Geometry: final body of the model. Coordinates: model frame, mm. Face numbers are marked on the shaded views. A direction names the side the tool comes from. Give positions to 0.01 mm unless a question says otherwise; leave off trailing zeros. Order: outer loops, then holes, each group sorted by start corner. A loop starts at its lowest first (then second) coordinate and runs counter-clockwise, first axis right, second up. Notation, with made-up numbers: M 84,1.25 L 119,1.25 A19 ccw 119,36.25 Z; hole C -13.5,89 d1. An arc over 180 degrees is marked long. Use CSV: the item, a comma, the result in double quotes.
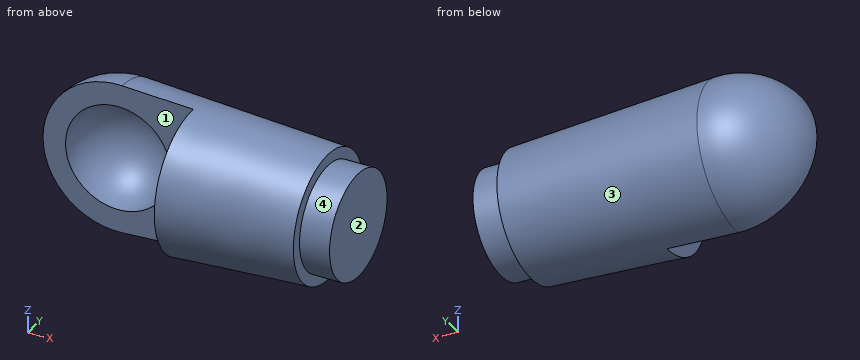
```python
from build123d import *

# Parameters (mm, degrees)
SKETCH2_W           = 100
SKETCH2_H           = 100
CUT_EXTRUDE1_DEPTH  = 62
SKETCH3_R           = 35
BOSS_EXTRUDE1_DEPTH = 20


with BuildPart() as part:
    # Sketch1 → Revolve1 (revolve)
    with BuildSketch(Plane(origin=(0, 0, 0), x_dir=(1, 0, 0), z_dir=(0, 1, 0)), mode=Mode.PRIVATE) as revolve1_sk:
        with BuildLine():
            Line((0, 0), (0, 42.5))
            Line((0, 42.5), (-137.299270073, 49.927007299))
            ThreePointArc((-137.299270073, 49.927007299), (-174.387232396, 36.297634195), (-190, 0))
            Line((-190, 0), (-175, 0))
            ThreePointArc((-175, 0), (-140, 35), (-105, 0))
            Line((-105, 0), (0, 0))
        make_face()
    revolve(revolve1_sk.sketch.rotate(Axis((-105, 0, 0), (1, 0, 0)), 180), axis=Axis((-105, 0, 0), (1, 0, 0)))

    # Sketch2 → Cut-Extrude1 (cut)
    with BuildSketch(Plane(origin=(0, 0, 0), x_dir=(1, 0, 0), z_dir=(0, 1, 0))):
        with Locations((-140, 0)):
            Rectangle(SKETCH2_W, SKETCH2_H)
    extrude(amount=-CUT_EXTRUDE1_DEPTH, mode=Mode.SUBTRACT)

    # Sketch3 → Boss-Extrude1 (add)
    with BuildSketch(Plane(origin=(0, 0, 0), x_dir=(0, 0, -1), z_dir=(1, 0, 0))):
        Circle(SKETCH3_R)
    extrude(amount=BOSS_EXTRUDE1_DEPTH)


solid = part.part
```
1. Pull-direction query (X, two-part tool) for the marked faces 3 and 4; classes: +X half, -X half, draft (parallel to the pull), parting line (faces both ways), or undercut.
Answer:
face 3,"+X half"
face 4,"draft"
2. Section A-A, the plane z = 0. Return the cut outline in (x, y), plus the area to 3 significant figures.
Answer:
outline,"M -190,0 L -175,0 A35 cw -105,0 L -90,0 L -90,-47.37 L 0,-42.5 L 0,-35 L 20,-35 L 20,35 L 0,35 L 0,42.5 L -137.3,49.93 A50 ccw Z"
area,"12,000 mm2"
3. Line query: line 1 (X direction, y = -18, z = 19); line 2 (X direction, y = 23, z = -24.5); line 3 (Z direction, x = -153.5, y = 20.5). Output: solid intervals per line, ascending.
Answer:
line 1,"-90 to 20"
line 2,"-177.02 to -149.79, -130.21 to 20"
line 3,"-43.56 to -24.95, 24.95 to 43.56"
4. Section C-C, the plane x = -153.5. Return the cut outline in (y, z), plus the area to 3 significant figures.
Answer:
outline,"M 0,-48.14 A48.14 ccw 0,48.14 L 0,32.29 A32.29 cw 0,-32.29 Z"
area,"2,000 mm2"
5. Reachability of the marked faces 1 and 2 from +Z, -Z, +X, -X, +Y, -Y: full face, straight path, thin tool, end or side. Return the list, or none.
Answer:
face 1,"+Z, -Z, -X, -Y"
face 2,"+Z, -Z, +X, +Y, -Y"
6. Section D-D, the plane x = -13. Return the cut outline in (y, z).
Answer:
outline,"C 0,0 d86.41"
7. Pin query (flat end, axial travel): pin 1 Ø5 at (x, y) = (-4, 23.5) entering from +Z; pin 2 Ø8 at (x, y) = (-14, 4) entering from -Z; pin 3 Ø14 at (y, z) = (-17.5, -16.5) entering from -X. Return the tip coordinate at first contact, or that it passes through.
Answer:
pin 1,"z = 37.21"
pin 2,"z = -43.4"
pin 3,"x = -90"
8. Section B-B, the plane x = -45.5. Return the cut outline in (y, z), plus the area to 3 significant figures.
Answer:
outline,"C 0,0 d89.92"
area,"6,350 mm2"
